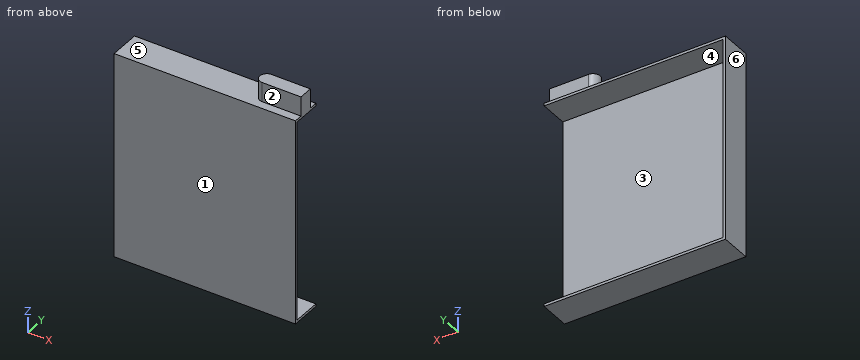
```python
from build123d import *

# Parameters (mm, degrees)
SKETCH_1_W      = 138
SKETCH_1_H      = 155
EXTRUDE_1_DEPTH = 22
SHELL_1_T       = 2
EXTRUDE_2_DEPTH = 15


with BuildPart() as part:
    # 草图1 → 凸台-拉伸1 (new body)
    with BuildSketch(Plane(origin=(0, 0, 0), x_dir=(1, 0, 0), z_dir=(0, 1, 0))):
        with Locations((69, -77.5)):
            Rectangle(SKETCH_1_W, SKETCH_1_H)
    extrude(amount=EXTRUDE_1_DEPTH)

    # 抽壳1
    shell_1_openings = [part.faces().sort_by_distance(p)[0] for p in [
        (138, 11, 77.5),
        (69, 22, 77.5),
    ]]
    offset(amount=SHELL_1_T, openings=shell_1_openings, kind=Kind.INTERSECTION)

    # 草图2 → 凸台-拉伸2 (add)
    with BuildSketch(Plane.XY.offset(157)):
        with BuildLine():
            Line((108, 15.5), (138, 15.5))
            Line((138, 15.5), (138, 4.5))
            Line((138, 4.5), (108, 4.5))
            ThreePointArc((108, 4.5), (102.5, 10), (108, 15.5))
        make_face()
    extrude(amount=EXTRUDE_2_DEPTH)


solid = part.part
```
Work out the finished part from the listing and answer in its coordinate system (mm). Face numbers are marked on the shaded views. A direction names the side the tool comes from. Give positions to 0.01 mm unless a question says otherwise; leave off trailing zeros. Order: outer loops, then holes, each group sorted by start corner. A loop starts at its lowest first (then second) coordinate and runs counter-clockwise, first axis right, second up. Notation, with made-up numbers: (35, 63.25) - (82, 63.25) arc R24 cw to (82, 77.25) - close; hole circle Ø7 at (59.25, 49). An arc over 180 degrees is marked (long way). One line per item, written item: value. Start each with the question number.
1. Each of these flat-tipped pins is pushed along its axis until it touches: pin 1 Ø8 at (x, z) = (69.5, 27.5) entering from +Y; pin 2 Ø6 at (y, z) = (19, 32.5) entering from +X; pin 3 Ø11 at (x, y) = (55.5, 7) entering from +Z. Where does it stop, or does it pass through?
2. Consider line 1 (Z direction, x = 107, y = 5.5); line 2 (Z direction, x = 124, y = 4); line 3 (Y direction, x = 130.5, z = 151.5). Determine where each line is inside the solid, lowest interval first.
3. For a pull along Z with two mould halves and no side action, classify the marked faces 3, 4, 5 and 6 as released by +Z, released by -Z, zero draft, split by the parting line, or undercut.
4. Section B-B, the plane x = 111.5 is taken. Write down the section's boundary in (y, z), then the cut area to 3 significant figures.
5. Which of the six approach directions +Z, -Z, +X, -X, +Y, -Y give full straight-line access (tool end or side, diameter ignored) to the marked faces 1 and 2?
6. Section A-A, the plane y = 10 is taken. Write down the section's boundary in (x, z), then the cut area to 3 significant figures.
7. Section C-C, the plane z = 66.5 is taken. Write down the section's boundary in (x, y).
8. Section D-D, the plane x = 96 is taken. Write down the section's boundary in (y, z), then the cut area to 3 significant figures.
Filled sheet:
1. pin 1: y = 0
1. pin 2: x = 0
1. pin 3: z = 157
2. line 1: -2 to 0, 155 to 172
2. line 2: -2 to 0, 155 to 157
2. line 3: -2 to 0
3. face 3: undercut
3. face 4: undercut
3. face 5: released by +Z
3. face 6: zero draft
4. outline: (-2, -2) - (22, -2) - (22, 0) - (0, 0) - (0, 155) - (22, 155) - (22, 157) - (15.5, 157) - (15.5, 172) - (4.5, 172) - (4.5, 157) - (-2, 157) - close
4. area: 571 mm²
5. face 1: +Z, -Z, +X, -X, -Y
5. face 2: +Z, +X, -X, -Y
6. outline: (-2, -2) - (138, -2) - (138, 0) - (0, 0) - (0, 155) - (138, 155) - (138, 172) - (102.5, 172) - (102.5, 157) - (-2, 157) - close
6. area: 1,400 mm²
7. outline: (-2, -2) - (138, -2) - (138, 0) - (0, 0) - (0, 22) - (-2, 22) - close
8. outline: (-2, -2) - (22, -2) - (22, 0) - (0, 0) - (0, 155) - (22, 155) - (22, 157) - (-2, 157) - close
8. area: 406 mm²
